Could you check a few things on this drawing? It's one solid part, dimensions in mm from its lowest x, y, z. A direction names the side the tool comes from. Round coordinates to 2 decimals unless told otherwise and drop trailing zeros. Write each loop counter-clockwise with the first axis right and the second up, starting at its lowest first coordinate (ties: lowest second). Pieces come first, ordered by that corner, then holes. Notation, with made-up numbers: (-3, 4.5) -> (32, 4.5) arc R20 ccw to (32, 42.5) -> close; hole circle Ø6 at (-20, -7.5). An arc over 180 degrees is marked (long way). Answer in a Markdown table with one row per item. Add a question column.
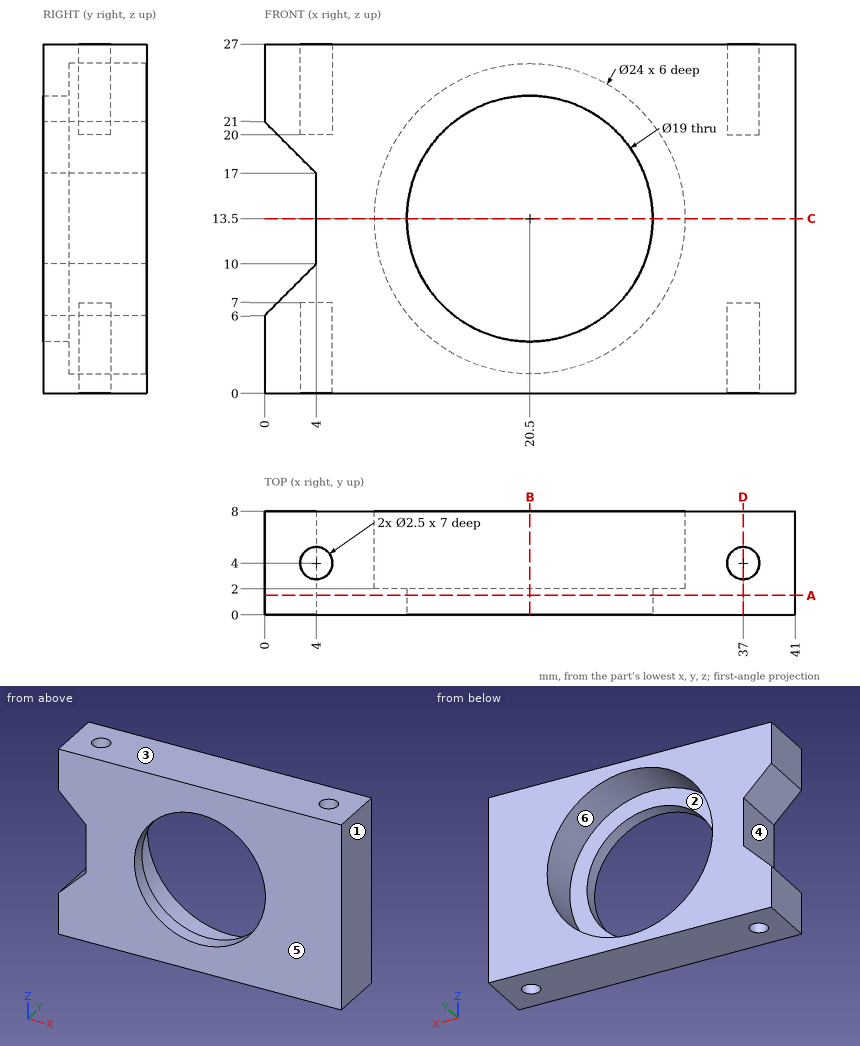
(1) Suppose I cut it at D-D, the plane x = 37. Please give me the cut outline in (y, z).
(2) If we mould it in two halves opening along Z, with no side actions, what happens to the marked faces 1, 2 and 3? For each: pulls with the +Z half, pulls with the -Z half, needs draft (parallel to the pull), parting line crosses it, or undercut.
(3) Suppose I cut it at A-A, the plane y = 1.5. Please give me the cut outline in (x, z), then the cut area to 3 significant figures.
(4) I need wall thicknesses on L1, parallel to Y at x = 37, z = 24.25; L2, parallel to X at y = 3.5, z = 4; L3, parallel to X at y = 4.2, z = 13.5. Which ranges of each line are inside material? Lowest first, please.
(5) Suppose I cut it at B-B, the plane x = 20.5. Please give me the cut outline in (y, z).
(6) Suppose I cut it at C-C, the plane z = 13.5. Please give me the cut outline in (x, y), then the cut area to 3 significant figures.
(7) On a 3-axis mill with a long thin cutter (end or side, diameter ignored), from which of +Z, -Z, +X, -X, +Y, -Y can I reach the whole of each face in a straight line? I mean the marked faces 4, 5 and 6. Say none if no direction works.
(8) For P1, Ø1.5, axis at x = 37, y = 4, coming from the -Z side; P2, Ø1.2, axis at x = 36.5, y = 4, coming from the +Z side, each with a flat end and sliding along its axis, tell me the tip position at first contact or that it passes through.
Response:
| question | item | result |
|---|---|---|
| 1 | outline | (0, 0) -> (2.75, 0) -> (2.75, 7) -> (5.25, 7) -> (5.25, 0) -> (8, 0) -> (8, 27) -> (5.25, 27) -> (5.25, 20) -> (2.75, 20) -> (2.75, 27) -> (0, 27) -> close |
| 2 | face 1 | needs draft |
| 2 | face 2 | undercut |
| 2 | face 3 | pulls with the +Z half |
| 3 | outline | (0, 0) -> (41, 0) -> (41, 27) -> (0, 27) -> (0, 21) -> (4, 17) -> (4, 10) -> (0, 6) -> close; hole circle Ø19 at (20.5, 13.5) |
| 3 | area | 779 mm² |
| 4 | L1 | 0 to 2.75, 5.25 to 8 |
| 4 | L2 | 0 to 2.85, 5.15 to 13.17, 27.83 to 35.85, 38.15 to 41 |
| 4 | L3 | 4 to 8.5, 32.5 to 41 |
| 5 | outline | (0, 0) -> (8, 0) -> (8, 1.5) -> (2, 1.5) -> (2, 4) -> (0, 4) -> close; (0, 23) -> (2, 23) -> (2, 25.5) -> (8, 25.5) -> (8, 27) -> (0, 27) -> close |
| 6 | outline | (4, 0) -> (11, 0) -> (11, 2) -> (8.5, 2) -> (8.5, 8) -> (4, 8) -> close; (30, 0) -> (41, 0) -> (41, 8) -> (32.5, 8) -> (32.5, 2) -> (30, 2) -> close |
| 6 | area | 114 mm² |
| 7 | face 4 | -X, +Y, -Y |
| 7 | face 5 | +Z, -Z, +X, -X, -Y |
| 7 | face 6 | +Y |
| 8 | P1 | z = 7 |
| 8 | P2 | z = 20 |
